Could you check a few things on this model? Use its own coordinates, in mm. A direction names the side the tool comes from. Coordinates: 2 decimals unless noted, no trailing zeros. Loops run counter-clockwise (first coordinate to the right, second up) from the corner with the lowest first, then second, coordinate; pieces in that order, holes last. Notation, with made-up numbers: (88, 30) - (114, 30) arc R25 ccw to (114, 66) - close; hole circle Ø7 at (68, 30). An arc over 180 degrees is marked (long way). One line per item, written item: value. Start each with the question number.
(1) If we section it at A-A on y = 0.55: Write out the boundary of the cut face in (x, z).
(2) On a 3-axis mill with a long thin cutter (end or side, diameter ignored), from which of +Z, -Z, +X, -X, +Y, -Y can I reach the whole of each face in a straight line? I mean faces 4 (the face through (65.1, 0, 25)), 5 (the face through (5.1, 0, 0)), 6 (the face through (3, 0, 22.505)). Say none if no direction works.
(3) If I drill on line 1 along X through (y, z) = (-1.1, -7), over which ranges is the centre line in solid material (lowest first)? Write a range as from..to.
(4) If we section it at B-B on z = -5: Write out the boundary of the cut face in (x, y).
(5) If we mould it in two halves opening along Z, with no side actions, what happens to faces 1 (the face through (65.1, 0, 0)), 2 (the face through (0, 0, -15)), 3 (the face through (35, 0, 27.005))? For each: pulls with the +Z half, pulls with the -Z half, needs draft (parallel to the pull), parting line crosses it, or undercut.
(6) I'm going to push flat-ended pins straight in: P1, Ø2.5, axis at x = 2.5, y = -0.5, coming from the -Z side; P2, Ø2, axis at y = -1, z = -26, coming from the +X side; P3, Ø1.5, axis at x = 67.5, y = -1, coming from the +Z side. Where does each tip first touch, or does it pass through?
```python
from build123d import *

# Parameters (mm, degrees)
SKETCH1_W           = 54.009051094
SKETCH1_H           = 5
BOSS_EXTRUDE1_DEPTH = 70.2
SKETCH5_W           = 5.1
SKETCH5_H           = 4.5
SKETCH5_H_2         = 15
CUT_EXTRUDE1_DEPTH  = 76.380928623


with BuildPart() as part:
    # Sketch1 → Boss-Extrude1 (new body)
    with BuildSketch(Plane(origin=(0, 0, 0), x_dir=(0, 0, -1), z_dir=(1, 0, 0))):
        Rectangle(SKETCH1_W, SKETCH1_H)
    extrude(amount=BOSS_EXTRUDE1_DEPTH)

    # Sketch5 → Cut-Extrude1 (cut, through all)
    with BuildSketch(Plane.XZ.offset(2.5)):
        with Locations((67.65, 24.754525547)):
            Rectangle(SKETCH5_W, SKETCH5_H)
        with Locations((67.65, -24.754525547)):
            Rectangle(SKETCH5_W, SKETCH5_H)
        with Locations((67.65, -0.004525547)):
            Rectangle(SKETCH5_W, SKETCH5_H_2)
        with Locations((2.55, -24.754525547)):
            Rectangle(SKETCH5_W, SKETCH5_H)
        with Locations((2.55, -0.004525547)):
            Rectangle(SKETCH5_W, SKETCH5_H_2)
        with Locations((2.55, 24.754525547)):
            Rectangle(SKETCH5_W, SKETCH5_H)
    extrude(amount=-CUT_EXTRUDE1_DEPTH, mode=Mode.SUBTRACT)


solid = part.part
```
Values:
1. outline: (0, -22.5) - (5.1, -22.5) - (5.1, -27) - (65.1, -27) - (65.1, -22.5) - (70.2, -22.5) - (70.2, -7.5) - (65.1, -7.5) - (65.1, 7.5) - (70.2, 7.5) - (70.2, 22.5) - (65.1, 22.5) - (65.1, 27) - (5.1, 27) - (5.1, 22.5) - (0, 22.5) - (0, 7.5) - (5.1, 7.5) - (5.1, -7.5) - (0, -7.5) - close
2. face 4: +Z, +X, +Y, -Y
2. face 5: -X, +Y, -Y
2. face 6: +Z, -X, +Y, -Y
3. line 1: x = 5.1..65.1
4. outline: (5.1, -2.5) - (65.1, -2.5) - (65.1, 2.5) - (5.1, 2.5) - close
5. face 1: undercut
5. face 2: needs draft
5. face 3: pulls with the +Z half
6. P1: stops at z = -22.5
6. P2: stops at x = 65.1
6. P3: stops at z = 22.5
